```python
from build123d import *

# Parameters (mm, degrees)
BOSS_EXTRUDE1_DEPTH         = 9.525
CUT_EXTRUDE1_REACH          = 312.187
SKETCH2_W                   = 19.05
SKETCH2_H                   = 6.35
FILLET1_R                   = 6.35
F_1_4_20_TAPPED_HOLE2_D     = 5.1054
F_1_4_20_TAPPED_HOLE2_DEPTH = 6.35
F_1_4_CLEARANCE_HOLE1_D     = 6.7564
F_1_4_CLEARANCE_HOLE1_DEPTH = 6.35
LPATTERN2_COUNT             = 24
LPATTERN2_PITCH             = 12.7


with BuildPart() as part:
    # Sketch1 → Boss-Extrude1 (new, symmetric)
    with BuildSketch(Plane(origin=(0, 0, 0), x_dir=(1, 0, 0), z_dir=(0, 1, 0))):
        Polygon((-56.762661738, -101.318299445), (16.262338262, -101.318299445), (16.262338262, 203.481700555), (-5.962661738, 203.481700555), (-5.962661738, 152.681700555), (-56.762661738, 152.681700555), align=None)
    extrude(amount=BOSS_EXTRUDE1_DEPTH, both=True)

    # Sketch2 → Cut-Extrude1 (cut, up to next)
    with BuildSketch(Plane.XY.offset(101.318299445), mode=Mode.PRIVATE) as cut_extrude1_sk1:
        with Locations((6.737338262, 0)):
            Rectangle(SKETCH2_W, SKETCH2_H)
    cut_extrude1_tool1 = extrude(cut_extrude1_sk1.sketch, amount=-CUT_EXTRUDE1_REACH, mode=Mode.PRIVATE) & part.part
    add(cut_extrude1_tool1.solids().sort_by_distance((6.737338, 0, 101.318299))[0], mode=Mode.SUBTRACT)

    # Fillet1
    fillet1_edges = [part.edges().sort_by_distance(p)[0] for p in [
        (-5.962661738, 0, -152.681700555),
    ]]
    fillet(fillet1_edges, radius=FILLET1_R)

    # 1/4-20 Tapped Hole2
    with Locations(Plane(origin=(0, 9.525, 0), x_dir=(1, 0, 0), z_dir=(0, 1, 0))):
        with Locations((9.912338262, 197.131700555)):
            f_1_4_20_tapped_hole2 = Hole(F_1_4_20_TAPPED_HOLE2_D / 2, depth=F_1_4_20_TAPPED_HOLE2_DEPTH)

    # 1/4 Clearance Hole1
    with Locations(Plane(origin=(0, -3.175, 0), x_dir=(1, 0, 0), z_dir=(0, 1, 0))):
        with Locations((9.912338262, 197.131700555)):
            f_1_4_clearance_hole1 = Hole(F_1_4_CLEARANCE_HOLE1_D / 2, depth=F_1_4_CLEARANCE_HOLE1_DEPTH)

    # LPattern2: 1/4-20 Tapped Hole2, 1/4 Clearance Hole1 ×24
    with Locations(*[(0, 0, i * LPATTERN2_PITCH) for i in range(1, LPATTERN2_COUNT)]):
        add(f_1_4_20_tapped_hole2, mode=Mode.SUBTRACT)
        add(f_1_4_clearance_hole1, mode=Mode.SUBTRACT)


solid = part.part
```
Input: part model. Units: mm. Frame: model coordinates. A direction names the side the tool comes from. Coordinates: 2 decimals unless noted, no trailing zeros. Loops run counter-clockwise (first coordinate to the right, second up) from the corner with the lowest first, then second, coordinate; pieces in that order, holes last. Notation, with made-up numbers: (59, 32.5) -> (75, 32.5) arc R22 cw to (75, 44.5) -> close; hole circle Ø1 at (45, 53). An arc over 180 degrees is marked (long way). Use a Markdown table: item, result.
1) Cut plane C-C (x = -33). Return the cut outline in (y, z) (3 decimals).
Results found:
| item | result |
|---|---|
| outline | (-9.525, -152.682) -> (9.525, -152.682) -> (9.525, 101.318) -> (-9.525, 101.318) -> close |
2) Cut plane B-B (y = -0.5). Return the cut outline in (x, z), then the cut area to 3 significant figures.
Results found:
| item | result |
|---|---|
| outline | (-56.76, -152.68) -> (-12.31, -152.68) arc R6.35 cw to (-5.96, -159.03) -> (-5.96, -203.48) -> (-2.79, -203.48) -> (-2.79, 101.32) -> (-56.76, 101.32) -> close |
| area | 13,900 mm2 |
3) Access query for faces 5 (the flat face through (16.262, 6, -49)), 6 (the flat face through (7, 3.175, -49)), 7 (the flat face through (-5.963, 0, -182)), 8 (the cylindrical face through (10.35, -6.39, -60.78)). Directions: +Z, -Z, +X, -X, +Y, -Y. A direction counts if a zero-diameter tool reaches every point of the face in a straight line with its end or side. Return the directions, or none.
Results found:
| item | result |
|---|---|
| face 5 | +Z, -Z, +X, +Y, -Y |
| face 6 | +Z, -Z, +X |
| face 7 | -Z, -X, +Y, -Y |
| face 8 | -Y |
4) Cut plane A-A (x = 3.5). Return the cut outline in (y, z) (3 decimals), then the cut area to 3 significant figures.
Results found:
| item | result |
|---|---|
| outline | (-9.525, -203.482) -> (-3.175, -203.482) -> (-3.175, 101.318) -> (-9.525, 101.318) -> close; (3.175, -203.482) -> (9.525, -203.482) -> (9.525, 101.318) -> (3.175, 101.318) -> close |
| area | 3,870 mm2 |
5) Contact query for flat-ended pins moving along their axis: pin 1 (6 mm diameter, centred on x = -47.5, y = -2, fed in from -Z); pin 2 (3 mm diameter, centred on x = 9.91, z = -184.43, fed in from +Y) (3 decimals); pin 3 (8 mm diameter, centred on x = 9.91, z = -82.83, fed in from -Y) (3 decimals); pin 4 (6 mm diameter, centred on x = 9.91, z = -19.33, fed in from -Y) (3 decimals). Output: stop coordinate, or through.
Results found:
| item | result |
|---|---|
| pin 1 | stops at z = -152.68 |
| pin 2 | passes through |
| pin 3 | stops at y = -9.525 |
| pin 4 | stops at y = 3.175 |
6) Material intervals for line 1 along Y through (x, z) = (6, -2.5) (3 decimals); line 2 along Z through (x, y) = (-53, 2.5); line 3 along X through (y, z) = (0.5, -60.5), sorted ascending. Write a range as from..to.
Results found:
| item | result |
|---|---|
| line 1 | y = -9.525..-3.175, 3.175..9.525 |
| line 2 | z = -152.68..101.32 |
| line 3 | x = -56.76..-2.79 |
7) Pull-direction query (Z, two-part tool) for faces 1 (the cylindrical face through (10.245, 6.306, -72.663)), 2 (the flat face through (-21, 0, 101.318)), 3 (the flat face through (-21, 9.525, -19)), 4 (the cylindrical face through (10.245, 6.306, -186.963)); classes: released by +Z, released by -Z, zero draft, split by the parting line, or undercut.
Results found:
| item | result |
|---|---|
| face 1 | undercut |
| face 2 | released by +Z |
| face 3 | zero draft |
| face 4 | undercut |
